from build123d import *

# Parameters (mm, degrees)
CYLINDER077_R               = 3.2
CYLINDER077_DEPTH           = 10
CYLINDER077_PLACEMENT_ANGLE = 25
CYLINDER012_R               = 1.8
CYLINDER012_DEPTH           = 15
CYLINDER012_PLACEMENT_ANGLE = 25
CYLINDER023_R               = 2.5
CYLINDER023_DEPTH           = 10
CYLINDER020_R               = 2.5
CYLINDER020_DEPTH           = 10
CYLINDER021_W               = 35
CYLINDER021_H               = 19
CYLINDER021_ANGLE           = 25
CYLINDER022_W               = 35
CYLINDER022_H               = 19
CYLINDER022_ANGLE           = 25
BOX029_W                    = 19
BOX029_H                    = 50
BOX029_DEPTH                = 4


with BuildPart() as cylinder073:
    # Cylinder077 → Cylinder077 (new body)
    with BuildSketch(Plane.XY):
        Circle(CYLINDER077_R)
    extrude(amount=CYLINDER077_DEPTH)


with BuildPart() as cylinder073_1:
    # Cylinder077 placement: moved
    add(cylinder073.part.moved(Location((177.5, 259.740915, 1.649137))).rotate(Axis((177.5, 259.740915, 1.649137), (-1, 0, 0)), CYLINDER077_PLACEMENT_ANGLE))


with BuildPart() as m2bolt:
    # Cylinder012 → Cylinder012 (new body)
    with BuildSketch(Plane.XY):
        Circle(CYLINDER012_R)
    extrude(amount=CYLINDER012_DEPTH)


with BuildPart() as m2bolt_1:
    # Cylinder012 placement: moved
    add(m2bolt.part.moved(Location((177.5, 263.58, 9.88971))).rotate(Axis((177.5, 263.58, 9.88971), (-1, 0, 0)), CYLINDER012_PLACEMENT_ANGLE))


with BuildPart() as m4s005:
    # Cylinder023 → Cylinder023 (new body)
    with BuildSketch(Plane(origin=(177.5, 240.5, 0), x_dir=(1, 0, 0), z_dir=(0, 0, 1))):
        Circle(CYLINDER023_R)
    extrude(amount=CYLINDER023_DEPTH)


with BuildPart() as m4lowcut002:
    # Cylinder020 → Cylinder020 (new body)
    with BuildSketch(Plane(origin=(177.5, 252.5, 0), x_dir=(1, 0, 0), z_dir=(0, 0, 1))):
        Circle(CYLINDER020_R)
    extrude(amount=CYLINDER020_DEPTH)

    # Fusion011: union m4s005
    add(m4s005.part)


with BuildPart() as cylinder021:
    # Cylinder021 → Cylinder021 (revolve)
    with BuildSketch(Plane(origin=(187, 283, 4), x_dir=(0, -1, 0), z_dir=(0, 0, -1))):
        with Locations((17.5, 9.5)):
            Rectangle(CYLINDER021_W, CYLINDER021_H)
    revolve(axis=Axis((187, 283, 4), (-1, 0, 0)), revolution_arc=CYLINDER021_ANGLE)


with BuildPart() as bottom004:
    # Cylinder022 → Cylinder022 (revolve)
    with BuildSketch(Plane(origin=(187, 292.5, 4), x_dir=(0, -1, 0), z_dir=(0, 0, -1))):
        with Locations((17.5, 9.5)):
            Rectangle(CYLINDER022_W, CYLINDER022_H)
    revolve(axis=Axis((187, 292.5, 4), (-1, 0, 0)), revolution_arc=CYLINDER022_ANGLE)

    # Cut018: cut Cylinder021
    add(cylinder021.part, mode=Mode.SUBTRACT)


with BuildPart() as bottommid001:
    # Box029 → Box029 (new body)
    with BuildSketch(Plane(origin=(168, 233.5, 4), x_dir=(1, 0, 0), z_dir=(0, 0, 1))):
        with Locations((9.5, 25)):
            Rectangle(BOX029_W, BOX029_H)
    extrude(amount=BOX029_DEPTH)

    # Fusion012: union bottom004
    add(bottom004.part)

    # Cut019: cut m4lowCut002
    add(m4lowcut002.part, mode=Mode.SUBTRACT)

    # Cut029: cut m2Bolt
    add(m2bolt_1.part, mode=Mode.SUBTRACT)

    # Cut060: cut Cylinder073
    add(cylinder073_1.part, mode=Mode.SUBTRACT)


solid = bottommid001.part
The listing builds one solid part. Answer for the finished solid, in the listing's coordinates (mm). Round coordinates to 2 decimals unless told otherwise and drop trailing zeros. Order: outer loops, then holes, each group sorted by start corner. A loop starts at its lowest first (then second) coordinate and runs counter-clockwise, first axis right, second up. Notation, with made-up numbers: (67, 51.5) -> (112, 51.5) arc R19 ccw to (112, 76.5) -> close; hole circle Ø7 at (52, 61). An arc over 180 degrees is marked (long way). Write each question's results on one line, items separated by ' | '. Start each with the question number.
Q1. Find section B-B (x = 177.5). Determine the outline of the cut face in (y, z).
Q2. Each of these flat-tipped pins is pushed along its axis until it touches: pin 1 (6 mm diameter, centred on x = 176, y = 264.5, fed in from +Z); pin 2 (10 mm diameter, centred on x = 174.5, y = 243, fed in from +Z); pin 3 (3 mm diameter, centred on x = 177.5, y = 252.5, fed in from +Z). Where does it stop, or does it pass through?
Q3. Straight lines are drawn through the part: probe 1 along X at (y, z) = (252.5, 5.85); probe 2 along Y at (x, z) = (177.5, 6.9); probe 3 along Y at (x, z) = (177.5, 5.75). For each, find the intervals that lie inside material, in ascending order. Write a range as from..to.
Q4. Find section C-C (x = 172.25). Determine the outline of the cut face in (y, z), then the cut area to 3 significant figures.
Q5. Find section A-A (y = 240.5). Determine the outline of the cut face in (x, z), then the cut area to 3 significant figures.
Q6. The mould has two halves that part along X. Classify faces 1 (the cylindrical face through (177.37, 259.97, 16.92)), 2 (the cylindrical face through (179.16, 265, 14.58)), 3 (the flat face through (187, 263, 6)): pulls with the +X half, pulls with the -X half, needs draft (parallel to the pull), parting line crosses it, or undercut.
Q7. Find section D-D (y = 249). Determine the outline of the cut face in (x, z).
Worked answers:
1) outline: (233.5, 4) -> (238, 4) -> (238, 8) -> (233.5, 8) -> close; (243, 4) -> (250, 4) -> (250, 8) -> (243, 8) -> close; (255, 4) -> (257.31, 4) -> (259.17, 8) -> (255, 8) -> close; (259.29, 15.06) -> (263.16, 13.25) -> (264.86, 16.89) -> (260.78, 18.79) arc R35 ccw to start; (264.37, 4) -> (292.5, 4) -> (268.12, 15.37) -> (266.42, 11.73) -> (274.42, 8) -> (266.23, 8) -> close
2) pin 1: stops at z = 18.46 | pin 2: stops at z = 8 | pin 3: passes through
3) probe 1: x = 168..175, 180..187 | probe 2: y = 233.5..238, 243..250, 255..258.66, 265.72..286.28 | probe 3: y = 233.5..238, 243..250, 255..258.12, 265.18..288.75
4) outline: (233.5, 4) -> (292.5, 4) -> (260.78, 18.79) arc R35 ccw to (259.29, 15.06) -> (274.42, 8) -> (233.5, 8) -> close | area: 304 mm2
5) outline: (168, 4) -> (175, 4) -> (175, 8) -> (168, 8) -> close; (180, 4) -> (187, 4) -> (187, 8) -> (180, 8) -> close | area: 56.0 mm2
6) face 1: needs draft | face 2: undercut | face 3: pulls with the +X half
7) outline: (168, 4) -> (187, 4) -> (187, 8) -> (168, 8) -> close
